from build123d import *

# Parameters (mm, degrees)
ESQUISSE2_W = 1
ESQUISSE2_H = 0.1
ESQUISSE3_W = 0.5
ESQUISSE3_H = 0.05
ESQUISSE4_W = 0.5
ESQUISSE4_H = 0.05
ESQUISSE5_W = 0.5
ESQUISSE5_H = 0.05


with BuildPart() as part:
    # Esquisse1 → Révolution1 (revolve)
    with BuildSketch(Plane.XY, mode=Mode.PRIVATE) as r_volution1_sk:
        Polygon((0, 0), (0, 1.75), (10, 1.75), (10.45, 1.3), (13, 1.5), (13.9, 0.6), (13.9, 0), align=None)
        Polygon((-1, 0), (0, 0), (0, 1.75), (0, 3), (-1, 3), align=None)
    revolve(r_volution1_sk.sketch.rotate(Axis((13.9, 0, 0), (-1, 0, 0)), 90), axis=Axis((13.9, 0, 0), (-1, 0, 0)))

    # Esquisse2 → End of connector (revolve, cut)
    with BuildSketch(Plane.XY, mode=Mode.PRIVATE) as end_of_connector_sk:
        with Locations((9.6, 1.7)):
            Rectangle(ESQUISSE2_W, ESQUISSE2_H)
    revolve(end_of_connector_sk.sketch.rotate(Axis((0, 0, 0), (1, 0, 0)), 90), axis=Axis((0, 0, 0), (1, 0, 0)), mode=Mode.SUBTRACT)

    # Esquisse3 → First connector separation (revolve, cut)
    with BuildSketch(Plane.XY, mode=Mode.PRIVATE) as first_connector_separation_sk:
        with Locations((9.35, 1.625)):
            Rectangle(ESQUISSE3_W, ESQUISSE3_H)
    revolve(first_connector_separation_sk.sketch.rotate(Axis((13.9, 0, 0), (1, 0, 0)), 90), axis=Axis((13.9, 0, 0), (1, 0, 0)), mode=Mode.SUBTRACT)

    # Esquisse4 → Second connector separation (revolve, cut)
    with BuildSketch(Plane.XY, mode=Mode.PRIVATE) as second_connector_separation_sk:
        with Locations((6.85, 1.725)):
            Rectangle(ESQUISSE4_W, ESQUISSE4_H)
    revolve(second_connector_separation_sk.sketch.rotate(Axis((13.9, 0, 0), (1, 0, 0)), 90), axis=Axis((13.9, 0, 0), (1, 0, 0)), mode=Mode.SUBTRACT)

    # Esquisse5 → Third connector sepatation (revolve, cut)
    with BuildSketch(Plane.XY, mode=Mode.PRIVATE) as third_connector_sepatation_sk:
        with Locations((4.35, 1.725)):
            Rectangle(ESQUISSE5_W, ESQUISSE5_H)
    revolve(third_connector_sepatation_sk.sketch.rotate(Axis((0, 0, 0), (-1, 0, 0)), 90), axis=Axis((0, 0, 0), (-1, 0, 0)), mode=Mode.SUBTRACT)


solid = part.part
Geometry: final body of the model. Coordinates: model frame, mm. A direction names the side the tool comes from. Give positions to 0.01 mm unless a question says otherwise; leave off trailing zeros. Write each loop counter-clockwise with the first axis right and the second up, starting at its lowest first coordinate (ties: lowest second). Pieces come first, ordered by that corner, then holes. Notation, with made-up numbers: (2, 19.5) -> (42, 19.5) arc R22 cw to (42, 55.5) -> close; hole circle Ø7 at (59.25, 18). An arc over 180 degrees is marked (long way). Answer in a Markdown table with one row per item.
(1) Ray query, line 1 along X through (y, z) = (-0.3, 1.95); line 2 along Z through (x, y) = (7, -0.8); line 3 along Z through (x, y) = (6.25, -1.15). Return the intervals inside material, ascending. Write a range as [from, to].
Answers below:
| item | result |
|---|---|
| line 1 | [-1, 0] |
| line 2 | [-1.5, 1.5] |
| line 3 | [-1.32, 1.32] |
(2) Draft query along X for faces 4 (the conical face through (11.743, 0.853, 1.112)), 5 (the flat face through (-1, 0, 0)), 6 (the cylindrical face through (2.08, 1.55, -0.81)). Return one class per face: +X half, -X half, draft (parallel to the pull), parting line (faces both ways), or undercut.
Answers below:
| item | result |
|---|---|
| face 4 | undercut |
| face 5 | -X half |
| face 6 | draft |
(3) Set-up query: faces 1 (the flat face through (13.9, 0, 0)), 2 (the cylindrical face through (9.354, -0.481, 1.526)), 3 (the cylindrical face through (9.854, -1.115, -1.216)). Return all of +Z, -Z, +X, -X, +Y, -Y with unobstructed straight access to the full face (end or side cutting, diameter ignored); none if empty.
Answers below:
| item | result |
|---|---|
| face 1 | +Z, -Z, +X, +Y, -Y |
| face 2 | none |
| face 3 | +X |
(4) Section query A-A on z = 2.4. Return loops of the section in (x, y), then the cut area to 3 significant figures.
Answers below:
| item | result |
|---|---|
| outline | (-1, -1.8) -> (0, -1.8) -> (0, 1.8) -> (-1, 1.8) -> close |
| area | 3.60 mm^2 |
(5) Section query C-C on y = -2.6. Return loops of the section in (x, z).
Answers below:
| item | result |
|---|---|
| outline | (-1, -1.5) -> (0, -1.5) -> (0, 1.5) -> (-1, 1.5) -> close |
(6) Section query B-B on x = 8.25. Return loops of the section in (y, z).
Answers below:
| item | result |
|---|---|
| outline | circle Ø3.5 at (0, 0) |
